Input: part model. Units: mm. Frame: model coordinates. Face numbers are marked on the shaded views. A direction names the side the tool comes from. Give positions to 0.01 mm unless a question says otherwise; leave off trailing zeros. Order: outer loops, then holes, each group sorted by start corner. A loop starts at its lowest first (then second) coordinate and runs counter-clockwise, first axis right, second up. Notation, with made-up numbers: (78, 87.25) - (118, 87.25) arc R21 ccw to (118, 111.25) - close; hole circle Ø9 at (10, 1). An arc over 180 degrees is marked (long way). Answer in a Markdown table with one row per item. Add a question column.
1. Ray query, line 1 (X direction, y = 2.8, z = 0) (3 decimals); line 2 (Y direction, x = -2, z = 1); line 3 (X direction, y = 20.05, z = 0) (3 decimals). Return the intervals inside material, ascending. Write a range as [from, to].
2. Access query for the marked faces 1, 2 and 3. Directions: +Z, -Z, +X, -X, +Y, -Y. A direction counts if a zero-diameter tool reaches every point of the face in a straight line with its end or side. Return the directions, or none.
3. Section query A-A on x = 10. Return loops of the section in (y, z) (3 decimals), and give its area (3 significant figures).
4. Mould query, pull axis X, two halves, no side actions, for the marked faces 4, 5 and 6. Classes: released by +X, released by -X, zero draft, split by the parting line, or undercut.
5. Section query B-B on y = 8.25. Return loops of the section in (x, z), and give its area (3 significant figures).
6. Section query C-C on x = -4. Return loops of the section in (y, z).
7. Contact query for flat-ended pins moving along their axis: pin 1 (3 mm diameter, centred on x = 8, z = -4.5, fed in from +Y); pin 2 (3 mm diameter, centred on y = 14, z = -6, fed in from -X); pin 3 (2 mm diameter, centred on x = 10, z = 0, fed in from -Y); pin 4 (2 mm diameter, centred on y = 2, z = 1, fed in from -X). Output: stop coordinate, or through.
8. Section query D-D on z = -3.75. Return loops of the section in (x, y), and give its area (3 significant figures).
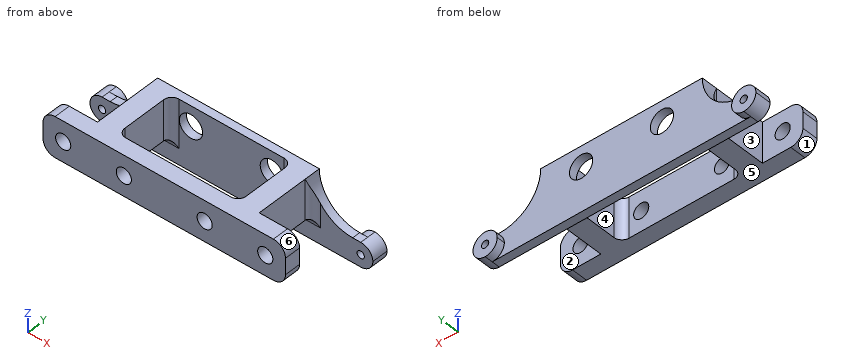
```python
from build123d import *

# Parameters (mm, degrees)
SKETCH1_W           = 60
SKETCH1_H           = 10
BOSS_EXTRUDE1_DEPTH = 4
SKETCH2_R           = 1.875
CUT_EXTRUDE1_DEPTH  = 31.6757233
SKETCH4_W           = 5
SKETCH4_H           = 10
BOSS_EXTRUDE2_DEPTH = 15
BOSS_EXTRUDE3_DEPTH = 4
SKETCH7_W           = 58
SKETCH7_H           = 6
CUT_EXTRUDE2_DEPTH  = 2
SKETCH9_W           = 40
SKETCH9_H           = 10
CUT_EXTRUDE3_DEPTH  = 2
CUT_EXTRUDE5_REACH  = 44.273
SKETCH10_R          = 2.875
FILLET1_R           = 10
FILLET2_R           = 3
FILLET3_R           = 2
SKETCH8_R           = 0.9
CUT_EXTRUDE4_DEPTH  = 44.301270189
FILLET4_R           = 2


# Some blends are built 0.0001 mm under size
with BuildPart() as part:
    # Sketch1 → Boss-Extrude1 (new body)
    with BuildSketch(Plane(origin=(0, 0, 0), x_dir=(1, 0, 0), z_dir=(0, 1, 0))):
        Rectangle(SKETCH1_W, SKETCH1_H)
    extrude(amount=BOSS_EXTRUDE1_DEPTH)

    # Sketch2 → Cut-Extrude1 (cut, through all)
    with BuildSketch(Plane(origin=(0, 4, 0), x_dir=(1, 0, 0), z_dir=(0, 1, 0))):
        with Locations(Location((-25, 0, 0), (0, 0, 270))):
            Circle(SKETCH2_R)
        with Locations(Location((-10, 0, 0), (0, 0, 270))):
            Circle(SKETCH2_R)
        with Locations(Location((10, 0, 0), (0, 0, 270))):
            Circle(SKETCH2_R)
        with Locations(Location((25, 0, 0), (0, 0, 270))):
            Circle(SKETCH2_R)
    extrude(amount=-CUT_EXTRUDE1_DEPTH, mode=Mode.SUBTRACT)

    # Sketch4 → Boss-Extrude2 (add)
    with BuildSketch(Plane(origin=(0, 4, 0), x_dir=(1, 0, 0), z_dir=(0, 1, 0))):
        with Locations((-17.5, 0)):
            Rectangle(SKETCH4_W, SKETCH4_H)
        with Locations((17.5, 0)):
            Rectangle(SKETCH4_W, SKETCH4_H)
    extrude(amount=BOSS_EXTRUDE2_DEPTH)

    # Sketch5 → Boss-Extrude3 (add)
    with BuildSketch(Plane(origin=(0, 19, 0), x_dir=(1, 0, 0), z_dir=(0, 1, 0))):
        Polygon((-20, -5), (20, -5), (20, 5), (35, 5), (35, 11), (-35, 11), (-35, 5), (-20, 5), align=None)
    extrude(amount=BOSS_EXTRUDE3_DEPTH)

    # Sketch7 → Cut-Extrude2 (cut)
    with BuildSketch(Plane(origin=(0, 23, 0), x_dir=(1, 0, 0), z_dir=(0, 1, 0))):
        with Locations((0, 8)):
            Rectangle(SKETCH7_W, SKETCH7_H)
    extrude(amount=-CUT_EXTRUDE2_DEPTH, mode=Mode.SUBTRACT)

    # Sketch9 → Cut-Extrude3 (cut)
    with BuildSketch(Plane(origin=(0, 23, 0), x_dir=(1, 0, 0), z_dir=(0, 1, 0))):
        Rectangle(SKETCH9_W, SKETCH9_H)
    extrude(amount=-CUT_EXTRUDE3_DEPTH, mode=Mode.SUBTRACT)

    # Sketch10 → Cut-Extrude5 (cut, up to next)
    with BuildSketch(Plane(origin=(0, 21, 0), x_dir=(1, 0, 0), z_dir=(0, 1, 0)), mode=Mode.PRIVATE) as cut_extrude5_sk1:
        with Locations(Location((-10, 0, 0), (0, 0, 270))):
            Circle(SKETCH10_R)
    cut_extrude5_tool1 = extrude(cut_extrude5_sk1.sketch, amount=-CUT_EXTRUDE5_REACH, mode=Mode.PRIVATE) & part.part
    # Sketch10 → Cut-Extrude5 (cut, up to next)
    with BuildSketch(Plane(origin=(0, 21, 0), x_dir=(1, 0, 0), z_dir=(0, 1, 0)), mode=Mode.PRIVATE) as cut_extrude5_sk2:
        with Locations(Location((10, 0, 0), (0, 0, 270))):
            Circle(SKETCH10_R)
    cut_extrude5_tool2 = extrude(cut_extrude5_sk2.sketch, amount=-CUT_EXTRUDE5_REACH, mode=Mode.PRIVATE) & part.part
    add(cut_extrude5_tool1.solids().sort_by_distance((-10, 21, 0))[0], mode=Mode.SUBTRACT)
    add(cut_extrude5_tool2.solids().sort_by_distance((10, 21, 0))[0], mode=Mode.SUBTRACT)

    # Fillet1
    fillet1_edges = [part.edges().sort_by_distance(p)[0] for p in [
        (20, 20, -5),
        (-20, 20, -5),
    ]]
    fillet(fillet1_edges, radius=FILLET1_R - 0.0001)  # a hair under: the kernel refuses the full size

    # Fillet2
    # the kernel refuses this fillet: 3 mm, written as the material it takes off along each edge
    with BuildSketch(Plane(origin=(30, -7.5, -5), x_dir=(-1, 0, 0), z_dir=(0, 1, 0)), Plane(origin=(-30, -7.5, 5), x_dir=(1, 0, 0), z_dir=(0, 1, 0)), Plane(origin=(-35, 11.5, -5), x_dir=(1, 0, 0), z_dir=(0, 1, 0)), Plane(origin=(35, 11.5, -11), x_dir=(-1, 0, 0), z_dir=(0, 1, 0))) as fillet2_piece_1:
        with BuildLine():
            CenterArc((FILLET2_R, FILLET2_R), FILLET2_R, 180, 90)
            Line((0, FILLET2_R), (0, 0))
            Line((0, 0), (FILLET2_R, 0))
        make_face()
    fillet2_piece_1_solid = extrude(amount=19, mode=Mode.PRIVATE)
    with BuildSketch(Plane(origin=(30, -7.5, 5), x_dir=(-1, 0, 0), z_dir=(0, 1, 0)), Plane(origin=(-30, -7.5, -5), x_dir=(1, 0, 0), z_dir=(0, 1, 0)), Plane(origin=(-35, 11.5, -11), x_dir=(1, 0, 0), z_dir=(0, 1, 0)), Plane(origin=(35, 11.5, -5), x_dir=(-1, 0, 0), z_dir=(0, 1, 0))) as fillet2_piece_2:
        with BuildLine():
            CenterArc((FILLET2_R, -FILLET2_R), FILLET2_R, 90, 90)
            Line((0, -FILLET2_R), (0, 0))
            Line((0, 0), (FILLET2_R, 0))
        make_face()
    fillet2_piece_2_solid = extrude(amount=19, mode=Mode.PRIVATE)
    with BuildSketch(Plane(origin=(-29, 30.5, -11), x_dir=(0, 0, 1), z_dir=(0, -1, 0)), Plane(origin=(29, 30.5, -11), x_dir=(1, 0, 0), z_dir=(0, -1, 0))) as fillet2_piece_3:
        with BuildLine():
            CenterArc((FILLET2_R, FILLET2_R), FILLET2_R, 180, 90)
            Line((0, FILLET2_R), (0, 0))
            Line((0, 0), (FILLET2_R, 0))
        make_face()
    fillet2_piece_3_solid = extrude(amount=9.5, mode=Mode.PRIVATE)
    with BuildSketch(Plane(origin=(-29, 21, -4.949883917), x_dir=(-0.9998604946563736, 0, -0.016703030428994153), z_dir=(0, 1, 0))) as fillet2_piece_4:
        with BuildLine():
            CenterArc((3.050527666, -2.999581484), FILLET2_R, 90.957057654, 90)
            Line((0.050946182, -3.049690575), (-0.249011967, -3.054701484))
            Line((-0.249011967, -3.054701484), (-0.299958148, -0.005010909))
            Line((-0.299958148, -0.005010909), (0.025007319, 0.298955906))
            ThreePointArc((0.025007319, 0.298955906), (0.99558669, 0.266550417), (2.995407665, 0.299958148))
            Line((2.995407665, 0.299958148), (3.000418574, 0))
        make_face()
    fillet2_piece_4_solid = extrude(amount=9.625290207, mode=Mode.PRIVATE)
    with BuildSketch(Plane(origin=(29, 21, -4.949883917), x_dir=(0.9998604946563736, 0, -0.01670303042899439), z_dir=(0, 1, 0))) as fillet2_piece_5:
        with BuildLine():
            CenterArc((3.050527666, 2.999581484), FILLET2_R, 179.042942346, 90)
            Line((0.050946182, 3.049690575), (-0.249011967, 3.054701484))
            Line((-0.249011967, 3.054701484), (-0.299958148, 0.005010909))
            Line((-0.299958148, 0.005010909), (0.025007319, -0.298955906))
            ThreePointArc((0.025007319, -0.298955906), (0.99558669, -0.266550417), (2.995407665, -0.299958148))
            Line((2.995407665, -0.299958148), (3.000418574, 0))
        make_face()
    fillet2_piece_5_solid = extrude(amount=9.625290207, mode=Mode.PRIVATE)
    add([fillet2_piece_1_solid, fillet2_piece_2_solid, fillet2_piece_3_solid, fillet2_piece_4_solid, fillet2_piece_5_solid], mode=Mode.SUBTRACT)

    # Fillet3
    fillet3_edges = [part.edges().sort_by_distance(p)[0] for p in [
        (-15, 4, 0),
        (-15, 19, 0),
        (15, 4, 0),
        (15, 19, 0),
    ]]
    fillet(fillet3_edges, radius=FILLET3_R)

    # Sketch8 → Cut-Extrude4 (cut, through all)
    with BuildSketch(Plane(origin=(0, 23, 0), x_dir=(1, 0, 0), z_dir=(0, 1, 0))):
        with Locations(Location((32, 8, 0), (0, 0, 270))):
            Circle(SKETCH8_R)
        with Locations(Location((-32, 8, 0), (0, 0, 270))):
            Circle(SKETCH8_R)
    extrude(amount=-CUT_EXTRUDE4_DEPTH, mode=Mode.SUBTRACT)

    # Fillet4
    fillet4_edges = [part.edges().sort_by_distance(p)[0] for p in [
        (-16.5, 19, -5),
        (16.5, 19, -5),
        (-20, 19, -5e-05),
        (20, 19, -5e-05),
    ]]
    fillet(fillet4_edges, radius=FILLET4_R - 0.0001)  # a hair under: the kernel refuses the full size


solid = part.part
```
Answer:
| question | item | result |
|---|---|---|
| 1 | line 1 | x = [-30, -26.875], [-23.125, -11.875], [-8.125, 8.125], [11.875, 23.125], [26.875, 30] |
| 1 | line 2 | y = [0, 4], [19, 21] |
| 1 | line 3 | x = [-21.34, -12.875], [-7.125, 7.125], [12.875, 21.34] |
| 2 | face 1 | -Z, -X, -Y |
| 2 | face 2 | +Z, -Z, +X |
| 2 | face 3 | +Z, -Z, -X |
| 3 | outline | (0, -5) - (4, -5) - (4, -1.875) - (0, -1.875) - close; (0, 1.875) - (4, 1.875) - (4, 5) - (0, 5) - close; (19, -11) - (21, -11) - (21, -2.875) - (19, -2.875) - close; (19, 2.875) - (21, 2.875) - (21, 5) - (19, 5) - close |
| 3 | area | 45.5 mm² |
| 4 | face 4 | undercut |
| 4 | face 5 | zero draft |
| 4 | face 6 | released by +X |
| 5 | outline | (-20, -5) - (-15, -5) - (-15, 5) - (-20, 5) - close; (15, -5) - (20, -5) - (20, 5) - (15, 5) - close |
| 5 | area | 100 mm² |
| 6 | outline | (0, -5) - (4, -5) - (4, 5) - (0, 5) - close; (19, -11) - (21, -11) - (21, 5) - (19, 5) - close |
| 7 | pin 1 | stops at y = 21 |
| 7 | pin 2 | stops at x = -20 |
| 7 | pin 3 | passes through |
| 7 | pin 4 | stops at x = -30 |
| 8 | outline | (-29.44, 0) - (29.44, 0) - (29.44, 4) - (20, 4) - (20, 17) arc R2 cw to (22, 19) - (25.16, 19) - (25.16, 21) - (-25.16, 21) - (-25.16, 19) - (-22, 19) arc R2 cw to (-20, 17) - (-20, 4) - (-29.44, 4) - close; hole (-15, 6) arc R2 ccw to (-13, 4) - (13, 4) arc R2 ccw to (15, 6) - (15, 17) arc R2 ccw to (13, 19) - (-13, 19) arc R2 ccw to (-15, 17) - close |
| 8 | area | 491 mm² |
